Work out the finished part from the listing and answer in its coordinate system (mm). A direction names the side the tool comes from. Coordinates: 2 decimals unless noted, no trailing zeros. Write each loop counter-clockwise with the first axis right and the second up, starting at its lowest first coordinate (ties: lowest second). Pieces come first, ordered by that corner, then holes. Notation, with made-up numbers: (26, 24) - (47, 24) arc R17 cw to (47, 28) - close; hole circle Ø5 at (65, 26). An arc over 180 degrees is marked (long way). One line per item, written item: value.
```python
from build123d import *

# Parameters (mm, degrees)
AUFSATZ_LINEAR_AUSTRAGEN1_DEPTH = 10
SKIZZE2_R                       = 1.5
SCHNITT_LINEAR_AUSTRAGEN1_DEPTH = 6
FASE1_SIZE                      = 2
VERRUNDUNG1_R                   = 2
VERRUNDUNG2_R                   = 4


with BuildPart() as part:
    # Skizze1 → Aufsatz-Linear austragen1 (new body, symmetric)
    with BuildSketch(Plane.XY):
        Polygon((-24, 0), (0, 0), (0, 5), (-8, 5), (-8, 41), (0, 41), (0, 45), (-12, 45), (-12, 5), (-24, 5), align=None)
    extrude(amount=AUFSATZ_LINEAR_AUSTRAGEN1_DEPTH, both=True)

    # Skizze2 → Schnitt-Linear austragen1 (cut, through all)
    with BuildSketch(Plane(origin=(0, 5, 0), x_dir=(1, 0, 0), z_dir=(0, 1, 0))):
        with Locations((-18, 0)):
            Circle(SKIZZE2_R)
    extrude(amount=-SCHNITT_LINEAR_AUSTRAGEN1_DEPTH, mode=Mode.SUBTRACT)

    # Fase1
    fase1_edges = [part.edges().sort_by_distance(p)[0] for p in [
        (-19.5, 5, 0),
    ]]
    chamfer(fase1_edges, length=FASE1_SIZE)

    # Verrundung1
    verrundung1_edges = [part.edges().sort_by_distance(p)[0] for p in [
        (-24, 5, 0),
        (-12, 5, 0),
        (0, 45, 0),
        (-8, 5, 0),
        (0, 5, 0),
    ]]
    fillet(verrundung1_edges, radius=VERRUNDUNG1_R)

    # Verrundung2
    verrundung2_edges = [part.edges().sort_by_distance(p)[0] for p in [
        (-12, 45, 0),
    ]]
    fillet(verrundung2_edges, radius=VERRUNDUNG2_R)


solid = part.part
```
Item 1: Section B-B, the plane z = 0 is taken. Determine the outline of the cut face in (x, y).
Evaluation:
outline: (-24, 0) - (-19.5, 0) - (-19.5, 3) - (-21.5, 5) - (-22, 5) arc R2 ccw to (-24, 3) - close; (-16.5, 0) - (0, 0) - (0, 3) arc R2 ccw to (-2, 5) - (-6, 5) arc R2 cw to (-8, 7) - (-8, 41) - (0, 41) - (0, 43) arc R2 ccw to (-2, 45) - (-8, 45) arc R4 ccw to (-12, 41) - (-12, 7) arc R2 cw to (-14, 5) - (-14.5, 5) - (-16.5, 3) - close
Item 2: Determine the mould class of faces 1 (the face through (-10, 18, -10)), 2 (the face through (-0.57, 44.4, 0.14)), 3 (the face through (-12, 0, 0)), 4 (the face through (-8, 24, 0)) for opening direction Y: +Y half, -Y half, draft (parallel to the pull), parting line (faces both ways), or undercut.
Evaluation:
face 1: draft
face 2: +Y half
face 3: -Y half
face 4: undercut
Item 3: Section D-D, the plane y = 29.5 is taken. Determine the outline of the cut face in (x, z), then the cut area to 3 significant figures.
Evaluation:
outline: (-12, -10) - (-8, -10) - (-8, 10) - (-12, 10) - close
area: 80.0 mm2
Item 4: Section C-C, the plane z = -5.5 is taken. Determine the outline of the cut face in (x, y).
Evaluation:
outline: (-24, 0) - (0, 0) - (0, 3) arc R2 ccw to (-2, 5) - (-6, 5) arc R2 cw to (-8, 7) - (-8, 41) - (0, 41) - (0, 43) arc R2 ccw to (-2, 45) - (-8, 45) arc R4 ccw to (-12, 41) - (-12, 7) arc R2 cw to (-14, 5) - (-22, 5) arc R2 ccw to (-24, 3) - close
Item 5: Given pin 1 (6 mm diameter, centred on y = 23, z = -4.5, fed in from +X); pin 2 (4 mm diameter, centred on x = -18, z = 0, fed in from +Y); pin 3 (10 mm diameter, centred on y = 19, z = -1.5, fed in from -X), each flat-ended and moving along its own axis, determine where each tip first touches the part or whether it passes through.
Evaluation:
pin 1: stops at x = -8
pin 2: stops at y = 3.5
pin 3: stops at x = -12
Item 6: Consider probe 1 along Y at (x, z) = (-3.5, 0.25); probe 2 along X at (y, z) = (0.85, 0); probe 3 along Z at (x, y) = (-18, 0.8). Determine where each line is inside the solid, lowest interval first.
Evaluation:
probe 1: y = 0 to 5, 41 to 45
probe 2: x = -24 to -19.5, -16.5 to 0
probe 3: z = -10 to -1.5, 1.5 to 10
Item 7: Section A-A, the plane x = -18 is taken. Determine the outline of the cut face in (y, z), then the cut area to 3 significant figures.
Evaluation:
outline: (0, -10) - (5, -10) - (5, -3.5) - (3, -1.5) - (0, -1.5) - close; (0, 1.5) - (3, 1.5) - (5, 3.5) - (5, 10) - (0, 10) - close
area: 81.0 mm2
Item 8: Which of the six approach directions +Z, -Z, +X, -X, +Y, -Y give full straight-line access (tool end or side, diameter ignored) to faces 5 (the face through (-12, 24, 0)), 6 (the face through (-0.57, 4.4, 0.14)), 7 (the face through (-10, 18, 10))?
Evaluation:
face 5: +Z, -Z, -X, +Y
face 6: +Z, -Z, +X
face 7: +Z, +X, -X, +Y, -Y
